The listing builds one solid part. Answer for the finished solid, in the listing's coordinates (mm). Face numbers are marked on the shaded views. A direction names the side the tool comes from. Coordinates: 2 decimals unless noted, no trailing zeros. Write each loop counter-clockwise with the first axis right and the second up, starting at its lowest first coordinate (ties: lowest second). Pieces come first, ordered by that corner, then holes. Notation, with made-up numbers: M 65,79.25 L 109,79.25 A31 cw 109,104.25 Z; hole C -3,47.5 d11. An arc over 180 degrees is marked long. Answer as a JSON object with one key per item and string values. Group by question number.
from build123d import *

# Parameters (mm, degrees)
F2_R     = 1.65
F2_R_2   = 1
F3_DEPTH = 25
F4_W     = 25
F4_H     = 26
F5_DEPTH = 18


with BuildPart() as f1:
    # F0 (on Front) → F1 (revolve)
    with BuildSketch(Plane.XZ):
        Polygon((0, 22), (0, 1), (42.5, 1), (42.5, 0), (52.5, 0), (69, 22), align=None)
    revolve(axis=Axis((0, 0, 11.5), (0, 0, 1)))

    # F2 (on face) → F3 (cut)
    with BuildSketch(Plane.XY.offset(22)):
        with Locations((-35, -22.5)):
            Circle(F2_R)
        with Locations((-12, -22.5)):
            Circle(F2_R)
        with Locations((18, -22.5)):
            Circle(F2_R)
        with Locations((44, -22.5)):
            Circle(F2_R_2)
    extrude(amount=-F3_DEPTH, mode=Mode.SUBTRACT)

    # F4 (on face) → F5 (cut)
    with BuildSketch(Plane.XY.offset(22)):
        with Locations((-18.5, 27)):
            Rectangle(F4_W, F4_H)
        with Locations((18.5, 27)):
            Rectangle(F4_W, F4_H)
    extrude(amount=-F5_DEPTH, mode=Mode.SUBTRACT)


solid = f1.part
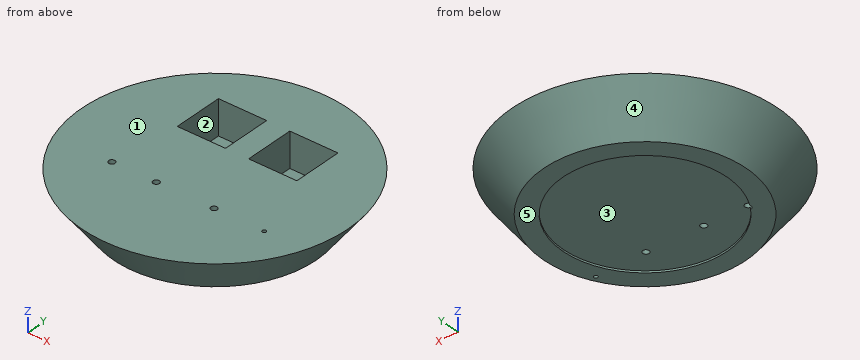
Item 1: Consider L1, parallel to Y at x = -12.5, z = 17.5; L2, parallel to X at y = -22, z = 18.75; L3, parallel to Y at x = -12, z = 7.25. Determine where each line is inside the solid, lowest interval first. Write a range as from..to.
Item 2: For a pull along X with two mould halves and no side action, classify the marked faces 3, 4 and 5 as +X half, -X half, draft (parallel to the pull), parting line (faces both ways), or undercut.
Item 3: Flat-ended cylindrical pins translate along their axes: pin 1 Ø1.2 at (x, y) = (44, -22.5) entering from +Z; pin 2 Ø7.5 at (x, y) = (17.5, 33.5) entering from +Z; pin 3 Ø9 at (x, z) = (-14.5, 11) entering from +Y; pin 4 Ø9 at (x, z) = (20.5, 17) entering from -Y. Find the tip coordinate at first contact, or state that the pin passes through.
Item 4: A tool of negligible diameter and unlimited length cuts with its end or side. For the marked faces 1 and 2, from which of +Z, -Z, +X, -X, +Y, -Y can it reach the whole face along a straight path? Write none if from no direction.
Item 5: A cutting plane is placed at A-A, the plane z = 14.5. Write down the section's boundary in (x, y) (3 decimals).
Answer:
{
 "1": {"L1": "-64.42..-24.07, -20.93..14, 40..64.42", "L2": "-62.82..-36.57, -33.43..-13.57, -10.43..16.43, 19.57..43.13, 44.87..62.82", "L3": "-56.68..-24.15, -20.85..14, 40..56.68"},
 "2": {"face 3": "undercut", "face 4": "parting line", "face 5": "draft"},
 "3": {"pin 1": "through", "pin 2": "z = 4", "pin 3": "y = 62.61", "pin 4": "y = -65.74"},
 "4": {"face 1": "+Z, +X, -X, +Y, -Y", "face 2": "+Z"},
 "5": {"outline": "C 0,0 d126.75; hole C -35,-22.5 d3.3; hole M -31,14 L -6,14 L -6,40 L -31,40 Z; hole C -12,-22.5 d3.3; hole M 6,14 L 31,14 L 31,40 L 6,40 Z; hole C 18,-22.5 d3.3; hole C 44,-22.5 d2"}
}
